Build history of the part. All positions in model axes, mm. A direction names the side the tool comes from. Give positions to 0.01 mm unless a question says otherwise; leave off trailing zeros. Loops run counter-clockwise (first coordinate to the right, second up) from the corner with the lowest first, then second, coordinate; pieces in that order, holes last.
1) Band-saw the part on C-C on y = 42.75. List the corners of the cut face in (x, z), then the cut area to 3 significant figures.
2) Band-saw the part on B-B on x = 2.5. State how many separate pieces and enclosed holes the cut face has, then the cut area to 3 significant figures.
3) Wall check: line 1 (Y direction, x = 0, z = 1.95); line 2 (X direction, y = -20, z = 5); line 3 (X direction, y = 0, z = 2.5). Give the ranges that are in metal, low to high.
4) Band-saw the part on A-A on y = 0. List the corners of the cut face in (x, z).
5) 3-axis set-ups, long thin cutter, end or side, ignore diameter. For faces 5 (the flat face through (0, -25.75, 5)), 6 (the flat face through (-27.75, 2, 3)), 7 (the flat face through (0, 36.75, 3)): which of +Z, -Z, +X, -X, +Y, -Y reach the whole face in a straight line?
6) Two-plate mould, pull along X, no slides. Class faces 1 (the cylindrical face through (-26.32, -26.25, 3.04)), 2 (the flat face through (-27, 0, 6)), 3 (the cylindrical face through (-24.85, 24.89, 4.48)), 4 (the cylindrical face through (-24.85, -24.89, 4.48)): +X half, -X half, draft (parallel to the pull), parting line (faces both ways), or undercut.
7) Flat gauge pins, fed straight in: P1, Ø3, axis at y = 12.5, z = 2.5, coming from the +X side; P2, Ø1.5, axis at y = 3.5, z = 4, coming from the -X side; P3, Ø2.5, axis at x = -22.08, y = 12.75, coming from the +Z side. Where does each tip first touch, or does it go through?
8) Band-saw the part on D-D on x = -24. List the corners of the cut face in (y, z), then the cut area to 3 significant figures.
```python
from build123d import *

# Parameters (mm, degrees)
SKETCH_W        = 55.5
SKETCH_H        = 55.5
SKETCH_R        = 22.75
PAD_DEPTH       = 6
SKETCH001_W     = 57.5
SKETCH001_H     = 8
PAD001_DEPTH    = 5
SKETCH002_W     = 30
SKETCH002_H     = 5
PAD002_DEPTH    = 20
FILLET_R        = 5
POCKET_DEPTH    = 6
FILLET001_R     = 9
FILLET002_R     = 7
CHAMFER_SIZE    = 3
SKETCH004_R     = 22.75
SKETCH004_R_2   = 22
PAD003_DEPTH    = 1.2
SKETCH005_W     = 51.5
SKETCH005_H     = 51.5
POCKET001_DEPTH = 3
SKETCH006_R     = 1
POCKET002_DEPTH = 6
FILLET003_R     = 1
FILLET004_R     = 1
FILLET005_R     = 3


with BuildPart() as part:
    # Sketch → Pad (new body)
    with BuildSketch(Plane.XY):
        Rectangle(SKETCH_W, SKETCH_H)
        Circle(SKETCH_R, mode=Mode.SUBTRACT)
    extrude(amount=PAD_DEPTH)

    # Sketch001 → Pad001 (new body)
    with BuildSketch(Plane(origin=(0, 27.75, 0), x_dir=(-1, 0, 0), z_dir=(0, 1, 0))):
        with Locations((0, 3)):
            Rectangle(SKETCH001_W, SKETCH001_H)
    extrude(amount=PAD001_DEPTH)

    # Sketch002 → Pad002 (new body)
    with BuildSketch(Plane(origin=(0, 32.75, 0), x_dir=(-1, 0, 0), z_dir=(0, 1, 0))):
        with Locations((0, 3)):
            Rectangle(SKETCH002_W, SKETCH002_H)
    extrude(amount=PAD002_DEPTH)

    # Fillet
    fillet_edges = [part.edges().sort_by_distance(p)[0] for p in [
        (-27.75, -27.75, 3),
        (27.75, -27.75, 3),
    ]]
    fillet(fillet_edges, radius=FILLET_R)

    # Sketch003 → Pocket (cut)
    with BuildSketch(Plane(origin=(0, 0, 0.5), x_dir=(1, 0, 0), z_dir=(0, 0, -1))):
        with BuildLine():
            ThreePointArc((-5, -36.75), (-11, -42.75), (-5, -48.75))
            Line((-5, -48.75), (5, -48.75))
            ThreePointArc((5, -48.75), (11, -42.75), (5, -36.75))
            Line((-5, -36.75), (5, -36.75))
        make_face()
    extrude(amount=-POCKET_DEPTH, mode=Mode.SUBTRACT)

    # Fillet001
    fillet001_edges = [part.edges().sort_by_distance(p)[0] for p in [
        (15, 52.75, 3),
        (-15, 52.75, 3),
    ]]
    fillet(fillet001_edges, radius=FILLET001_R)

    # Fillet002
    fillet002_edges = [part.edges().sort_by_distance(p)[0] for p in [
        (15, 32.75, 3),
        (-15, 32.75, 3),
    ]]
    fillet(fillet002_edges, radius=FILLET002_R)

    # Chamfer
    chamfer_edges = [part.edges().sort_by_distance(p)[0] for p in [
        (-28.75, 32.75, 3),
        (28.75, 32.75, 3),
    ]]
    chamfer(chamfer_edges, length=CHAMFER_SIZE)

    # Sketch004 → Pad003 (new body)
    with BuildSketch(Plane(origin=(0, 0, 0), x_dir=(1, 0, 0), z_dir=(0, 0, -1))):
        Circle(SKETCH004_R)
        Circle(SKETCH004_R_2, mode=Mode.SUBTRACT)
    extrude(amount=-PAD003_DEPTH)

    # Sketch005 → Pocket001 (cut)
    with BuildSketch(Plane.XY.offset(6)):
        Rectangle(SKETCH005_W, SKETCH005_H)
    extrude(amount=-POCKET001_DEPTH, mode=Mode.SUBTRACT)

    # Sketch006 → Pocket002 (cut)
    with BuildSketch(Plane.XY.offset(3)):
        with Locations((-22.083648, 12.75)):
            Circle(SKETCH006_R)
        with Locations((22.083648, 12.75)):
            Circle(SKETCH006_R)
        with Locations((-12.75, -22.083648)):
            Circle(SKETCH006_R)
    extrude(amount=-POCKET002_DEPTH, mode=Mode.SUBTRACT)

    # Fillet003
    fillet003_edges = [part.edges().sort_by_distance(p)[0] for p in [
        (0, 48.75, 5.5),
    ]]
    fillet(fillet003_edges, radius=FILLET003_R)

    # Fillet004
    fillet004_edges = [part.edges().sort_by_distance(p)[0] for p in [
        (0, 36.75, 0.5),
    ]]
    fillet(fillet004_edges, radius=FILLET004_R)

    # Fillet005
    fillet005_edges = [part.edges().sort_by_distance(p)[0] for p in [
        (-25.75, -25.75, 4.5),
        (25.75, -25.75, 4.5),
        (25.75, 25.75, 4.5),
        (-25.75, 25.75, 4.5),
    ]]
    fillet(fillet005_edges, radius=FILLET005_R)


solid = part.part
```
Findings below:
1. outline: (-15, 0.5) - (-12, 0.5) arc R1 ccw to (-11, 1.5) - (-11, 4.5) arc R1 ccw to (-12, 5.5) - (-15, 5.5) - close; (11, 1.5) arc R1 ccw to (12, 0.5) - (15, 0.5) - (15, 5.5) - (12, 5.5) arc R1 ccw to (11, 4.5) - close
1. area: 39.1 mm2
2. separate pieces: 3
2. enclosed holes: 0
2. area: 124 mm2
3. line 1: y = -27.75 to -22.75, 22.75 to 36.75, 48.75 to 52.75
3. line 2: x = -27.75 to -25.75, 25.75 to 27.75
3. line 3: x = -27.75 to -22.75, 22.75 to 27.75
4. outline: (-27.75, 0) - (-22, 0) - (-22, 1.2) - (-22.75, 1.2) - (-22.75, 3) - (-25.75, 3) - (-25.75, 6) - (-27.75, 6) - close; (22, 0) - (27.75, 0) - (27.75, 6) - (25.75, 6) - (25.75, 3) - (22.75, 3) - (22.75, 1.2) - (22, 1.2) - close
5. face 5: +Z
5. face 6: +Z, -Z, -X, -Y
5. face 7: +Z, -Z
6. face 1: -X half
6. face 2: draft
6. face 3: undercut
6. face 4: undercut
7. P1: stops at x = 27.75
7. P2: stops at x = -27.75
7. P3: stops at z = 3
8. outline: (-27.59, 0) - (27.75, 0) - (27.75, -1) - (32.75, -1) - (32.75, 7) - (27.75, 7) - (27.75, 6) - (25.48, 6) - (25.48, 3) - (-25.48, 3) - (-25.48, 6) - (-27.59, 6) - close
8. area: 219 mm2
